```python
from build123d import *

# Parameters (mm, degrees)
F0_R     = 3.875
F1_DEPTH = 3.4
F0_R_2   = 7
F2_DEPTH = 0.6
F0_R_3   = 11.5
F3_DEPTH = 2
F4_T     = 1


# Not quite as in the source:
# - a shell that OpenCascade refuses in one call is made with other operations: the cavity is built on its own and cut out


with BuildPart() as f1:
    # F0 (on Top) → F1 (new body)
    with BuildSketch(Plane.XY):
        Circle(F0_R)
    extrude(amount=F1_DEPTH)

    # F0 (on Top) → F2 (join)
    with BuildSketch(Plane.XY):
        Circle(F0_R_2)
        Circle(F0_R, mode=Mode.SUBTRACT)
    extrude(amount=F2_DEPTH)

    # F0 (on Top) → F3 (join)
    with BuildSketch(Plane.XY):
        Circle(F0_R_3)
        Circle(F0_R_2, mode=Mode.SUBTRACT)
        Circle(F0_R_2)
        Circle(F0_R, mode=Mode.SUBTRACT)
        Circle(F0_R)
    extrude(amount=-F3_DEPTH)

    # F4: shell of thickness 1, made by hand


with BuildPart() as f4_core1:
    # F4_t2: copy of F1
    add(f1.part)

    # the walls: a layer under each face that stays
    f4_faces = [f4_core1.faces().sort_by_distance(p)[0] for p in [
        (-11.5, 0, -1),
        (-7.6666666667, -7.6666666667, 0),
        (0, 0, -2),
        (-7, 0, 0.3),
        (-4.6666666667, -4.6666666667, 0.6),
        (-3.875, 0, 2),
    ]]
    thicken(f4_faces, amount=-F4_T, mode=Mode.SUBTRACT)

    # F4_s3 → F4_t4 (revolve, cut)
    with BuildSketch(Plane.XZ):
        Polygon((7.01, 0.01), (7, -1), (6, -1), (6, 0), align=None)
    revolve(axis=Axis((0, 0, 0), (0, 0, 1)), mode=Mode.SUBTRACT)

    # F4_s5 → F4_t6 (revolve, cut)
    with BuildSketch(Plane.XZ):
        Polygon((3.885, 0.61), (3.875, -0.4), (2.875, -0.4), (2.875, 0.6), align=None)
    revolve(axis=Axis((0, 0, 0.6), (0, 0, 1)), mode=Mode.SUBTRACT)


with BuildPart() as f1_1:
    add(f1.part)

    # what is left inside the walls is the cavity
    f4_cavity = [f4_core1.part.solids().sort_by_distance(p)[0] for p in [
        (0, -2, -0.99),
    ]]
    add(f4_cavity, mode=Mode.SUBTRACT)


solid = f1_1.part
```
Verification items for the finished model (mm, model axes). A direction names the side the tool comes from. Coordinates: 2 decimals unless noted, no trailing zeros. Loops run counter-clockwise (first coordinate to the right, second up) from the corner with the lowest first, then second, coordinate; pieces in that order, holes last. Notation, with made-up numbers: (-32.75, -34) -> (13.25, -34) arc R26 ccw to (13.25, -8) -> close; hole circle Ø10 at (35.25, -5.75). An arc over 180 degrees is marked (long way). Answer in a Markdown table with one row per item. Add a question column.
1. Section check A-A, the plane y = 0. Enter the section's corners in (x, z) (3 decimals).
2. Section check D-D, the plane x = 5. Enter the section's corners in (y, z).
3. Access from +Z, -Z, +X, -X, +Y, -Y to the whole of each face (thin tool, end or side, straight path). Record for faces 1 (the face through (0, -8, 0)), 2 (the face through (-1, 3, 3.4)), 3 (the face through (-5.994, 0.264, -0.696)).
4. Section check C-C, the plane z = 0.95. Enter the section's corners in (x, y) (3 decimals), then the cut area to 3 significant figures.
5. Material ranges on probe 1 along Z at (x, y) = (-1.5, 4.75); probe 2 along Z at (x, y) = (8.5, -4.5); probe 3 along Y at (x, z) = (0, -0.7), recorded low to high. Write a range as [from, to].
6. Depth check by flat-ended pin: P1, Ø2, axis at y = 4, z = 0, coming from the -X side; P2, Ø6, axis at x = 4.5, y = 8, coming from the +Z side; P3, Ø3, axis at x = -5, z = -1, coming from the +Y side. Enter the tip coordinate at first touch or a pass-through.
7. Draft check along Y on faces 4 (the face through (3, 1, -0.4)), 5 (the face through (3, -3, 0.6)), 6 (the face through (6.466, -2.681, 0.296)), 7 (the face through (-0.37, 2.85, 1.47)). Enter one of: +Y half, -Y half, draft (parallel to the pull), parting line (faces both ways), or undercut.
Derived:
| question | item | result |
|---|---|---|
| 1 | outline | (-11.5, -2) -> (11.5, -2) -> (11.5, 0) -> (7, 0) -> (7, 0.6) -> (3.875, 0.6) -> (3.875, 3.4) -> (2.875, 3.4) -> (2.875, -0.4) -> (6, -0.4) -> (6, -1) -> (-6, -1) -> (-6, -0.4) -> (-2.875, -0.4) -> (-2.875, 3.4) -> (-3.875, 3.4) -> (-3.875, 0.6) -> (-7, 0.6) -> (-7, 0) -> (-11.5, 0) -> close |
| 2 | outline | (-10.36, -2) -> (10.36, -2) -> (10.36, 0) -> (4.9, 0) -> (4.9, 0.6) -> (-4.9, 0.6) -> (-4.9, 0) -> (-10.36, 0) -> close; hole (-3.32, -1) -> (3.32, -1) -> (3.32, -0.4) -> (-3.32, -0.4) -> close |
| 3 | face 1 | +Z |
| 3 | face 2 | +Z, +X, -X, +Y, -Y |
| 3 | face 3 | none |
| 4 | outline | circle Ø7.75 at (0, 0); hole circle Ø5.75 at (0, 0) |
| 4 | area | 21.2 mm² |
| 5 | probe 1 | z = [-2, -1], [-0.4, 0.6] |
| 5 | probe 2 | z = [-2, 0] |
| 5 | probe 3 | y = [-11.5, -6], [6, 11.5] |
| 6 | P1 | stops at x = -11.1 |
| 6 | P2 | stops at z = 0.6 |
| 6 | P3 | stops at y = 10.95 |
| 7 | face 4 | undercut |
| 7 | face 5 | draft |
| 7 | face 6 | parting line |
| 7 | face 7 | undercut |
